The model under review builds one solid part; all positions refer to its coordinate system, in mm. Face numbers are marked on the shaded views. Give positions to 0.01 mm unless a question says otherwise; leave off trailing zeros. Loops run counter-clockwise (first coordinate to the right, second up) from the corner with the lowest first, then second, coordinate; pieces in that order, holes last. Notation, with made-up numbers: (33, 6) - (78, 6) arc R13 ccw to (78, 25) - close; hole circle Ø11 at (-26, 37.5). An arc over 180 degrees is marked (long way). Return JSON: item names as keys, results as strings. Group by question number.
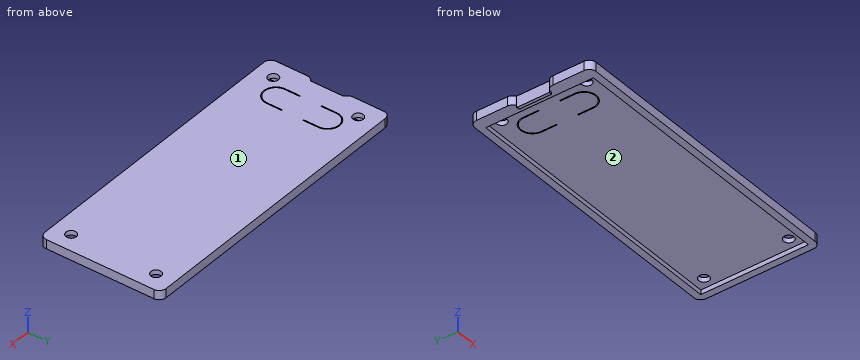
from build123d import *

# Parameters (mm, degrees)
SKETCH1_W           = 98
SKETCH1_H           = 40
BODY_DEPTH          = 3
SKETCH2_W           = 2.25
SKETCH2_H           = 10.5
CUT_EXTRUDE1_DEPTH  = 106.891453857
FILLET2_R           = 2.25
FILLET1_R           = 2.25
BOSS_EXTRUDE4_DEPTH = 3.7
SKETCH7_W           = 91.75
SKETCH7_H           = 35.5
OLED_RECESS_DEPTH   = 1.5
SKETCH9_R           = 1.7
CUT_EXTRUDE5_DEPTH  = 106.913596861


with BuildPart() as part:
    # Sketch1 → body (new body)
    with BuildSketch(Plane.XY):
        with Locations((49, 20)):
            Rectangle(SKETCH1_W, SKETCH1_H)
    extrude(amount=BODY_DEPTH)

    # Sketch2 → Cut-Extrude1 (cut, through all)
    with BuildSketch(Plane.XY.offset(3)):
        with Locations((1.125, 20)):
            Rectangle(SKETCH2_W, SKETCH2_H)
    extrude(amount=-CUT_EXTRUDE1_DEPTH, mode=Mode.SUBTRACT)

    # Fillet2
    fillet2_edges = [part.edges().sort_by_distance(p)[0] for p in [
        (0, 14.75, 1.5),
        (0, 25.25, 1.5),
    ]]
    fillet(fillet2_edges, radius=FILLET2_R - 0.0001)  # a hair under: the kernel refuses the full size

    # Fillet1
    fillet1_edges = [part.edges().sort_by_distance(p)[0] for p in [
        (0, 40, 1.5),
        (98, 40, 1.5),
        (98, 0, 1.5),
        (0, 0, 1.5),
    ]]
    fillet(fillet1_edges, radius=FILLET1_R)

    # Sketch6 → Boss-Extrude4 (add)
    with BuildSketch(Plane.XY.offset(3)):
        with BuildLine():
            Line((1.25, 25.484435563), (1.25, 14.515564437))
            ThreePointArc((1.25, 14.515564437), (1.736443763, 14.69060722), (2.25, 14.75))
            Line((2.25, 14.75), (2.25, 25.25))
            ThreePointArc((2.25, 25.25), (1.736443763, 25.30939278), (1.25, 25.484435563))
        make_face()
    extrude(amount=-BOSS_EXTRUDE4_DEPTH)

    # Sketch7 → oled-recess (cut)
    with BuildSketch(Plane(origin=(0, 0, 0), x_dir=(-1, 0, 0), z_dir=(0, 0, -1))):
        with Locations((-49.875, 20)):
            Rectangle(SKETCH7_W, SKETCH7_H)
    extrude(amount=-OLED_RECESS_DEPTH, mode=Mode.SUBTRACT)

    # Sketch9 → Cut-Extrude5 (cut, through all)
    with BuildSketch(Plane.XY.offset(3)):
        with Locations((6, 34)):
            Circle(SKETCH9_R)
        with Locations((92.25, 34)):
            Circle(SKETCH9_R)
        with Locations((6, 6)):
            Circle(SKETCH9_R)
        with Locations((92.25, 6)):
            Circle(SKETCH9_R)
        with BuildLine():
            Line((8, 28.5), (8, 23.5))
            Line((8, 23.5), (8.3, 23.5))
            Line((8.3, 23.5), (8.3, 28.5))
            ThreePointArc((8.3, 28.5), (12, 32.2), (15.7, 28.5))
            Line((15.7, 28.5), (15.7, 23.5))
            Line((15.7, 23.5), (16, 23.5))
            Line((16, 23.5), (16, 28.5))
            ThreePointArc((16, 28.5), (12, 32.5), (8, 28.5))
        make_face()
        with BuildLine():
            Line((15.7, 16.5), (16, 16.5))
            Line((16, 16.5), (16, 11.5))
            ThreePointArc((16, 11.5), (12, 7.5), (8, 11.5))
            Line((8, 11.5), (8, 16.5))
            Line((8, 16.5), (8.3, 16.5))
            Line((8.3, 16.5), (8.3, 11.5))
            ThreePointArc((8.3, 11.5), (12, 7.8), (15.7, 11.5))
            Line((15.7, 11.5), (15.7, 16.5))
        make_face()
    extrude(amount=-CUT_EXTRUDE5_DEPTH, mode=Mode.SUBTRACT)


solid = part.part
Item 1: Mouldability with a two-part tool opening along Y and no side actions: class the marked faces 1 and 2 as +Y half, -Y half, draft (parallel to the pull), parting line (faces both ways), or undercut.
Item 2: For P1, Ø0.8, axis at y = 19, z = -0.5, coming from the +X side; P2, Ø5, axis at x = 29, y = 4, coming from the -Z side; P3, Ø2, axis at x = 6, y = 34, coming from the +Z side; P4, Ø0.8, axis at y = 25, z = 2, coming from the -X side, all flat-tipped, find the tip position at first contact; note any pin that passes through.
Item 3: Take a section at B-B (y = 34). State the section outline as (x, z) points.
Item 4: For L1, parallel to Y at x = 92.25, z = 2.45; L2, parallel to X at y = 12, z = 2.7; L3, parallel to Y at x = 52, z = 0.6, list the stretches that pass through material, from the lowest coordinate up. Write a range as from..to.
Item 5: Take a section at C-C (z = 2.3). State how many separate pieces and enclosed holes the cut face has, then the cut area to 3 significant figures.
Item 6: Take a section at D-D (y = 17.5). State the section outline as (x, z) points, then the cut area to 3 significant figures.
Item 7: Take a section at A-A (x = 92.25). State the section outline as (y, z) points.
Check sheet entries:
{
 "1": {"face 1": "draft", "face 2": "undercut"},
 "2": {"P1": "stops at x = 2.25", "P2": "stops at z = 0", "P3": "passes through", "P4": "stops at x = 1.25"},
 "3": {"outline": "(0, 0) - (4, 0) - (4, 1.5) - (4.3, 1.5) - (4.3, 3) - (0, 3) - close; (7.7, 1.5) - (90.55, 1.5) - (90.55, 3) - (7.7, 3) - close; (93.95, 1.5) - (95.75, 1.5) - (95.75, 0) - (98, 0) - (98, 3) - (93.95, 3) - close"},
 "4": {"L1": "y = 0..4.3, 7.7..32.3, 35.7..40", "L2": "x = 0..8, 8.3..15.7, 16..98", "L3": "y = 0..2.25, 37.75..40"},
 "5": {"separate pieces": "1", "enclosed holes": "6", "area": "3,850 mm^2"},
 "6": {"outline": "(1.25, -0.7) - (2.25, -0.7) - (2.25, 0) - (4, 0) - (4, 1.5) - (95.75, 1.5) - (95.75, 0) - (98, 0) - (98, 3) - (1.25, 3) - close", "area": "153 mm^2"},
 "7": {"outline": "(0, 0) - (2.25, 0) - (2.25, 1.5) - (4.3, 1.5) - (4.3, 3) - (0, 3) - close; (7.7, 1.5) - (32.3, 1.5) - (32.3, 3) - (7.7, 3) - close; (35.7, 1.5) - (37.75, 1.5) - (37.75, 0) - (40, 0) - (40, 3) - (35.7, 3) - close"}
}
